from build123d import *

# Parameters (mm, degrees)
SKETCH1_R           = 25
SKETCH1_R_2         = 22.5
BOSS_EXTRUDE1_DEPTH = 130
SKETCH2_R           = 25
BOSS_EXTRUDE2_DEPTH = 5
BOSS_EXTRUDE3_DEPTH = 3
SKETCH4_R           = 2
BOSS_EXTRUDE4_DEPTH = 10


with BuildPart() as part:
    # Sketch1 → Boss-Extrude1 (new body)
    with BuildSketch(Plane(origin=(0, 0, 0), x_dir=(1, 0, 0), z_dir=(0, 1, 0))):
        Circle(SKETCH1_R)
        Circle(SKETCH1_R_2, mode=Mode.SUBTRACT)
    extrude(amount=BOSS_EXTRUDE1_DEPTH)

    # Sketch2 → Boss-Extrude2 (add)
    with BuildSketch(Plane.XZ):
        Circle(SKETCH2_R)
    extrude(amount=-BOSS_EXTRUDE2_DEPTH)

    # Sketch3 → Boss-Extrude3 (add)
    with BuildSketch(Plane(origin=(0, 130, 0), x_dir=(1, 0, 0), z_dir=(0, 1, 0))):
        with BuildLine():
            ThreePointArc((-2.5, 24.874685928), (-1.251569376, 24.968651828), (0, 25))
            Line((0, 25), (0, 40))
            Line((0, 40), (-2.5, 40))
            Line((-2.5, 40), (-2.5, 24.874685928))
        make_face()
        with BuildLine():
            Line((0, 40), (0, 25))
            ThreePointArc((0, 25), (1.251569376, 24.968651828), (2.5, 24.874685928))
            Line((2.5, 24.874685928), (2.5, 40))
            Line((2.5, 40), (0, 40))
        make_face()
    extrude(amount=-BOSS_EXTRUDE3_DEPTH)

    # Sketch4 → Boss-Extrude4 (add)
    with BuildSketch(Plane.XZ.offset(-127)):
        with Locations((0, -38)):
            Circle(SKETCH4_R)
    extrude(amount=BOSS_EXTRUDE4_DEPTH)


solid = part.part
Source: CAD feature listing. Evaluate the final solid. Frame: model axes, mm. A direction names the side the tool comes from. Give positions to 0.01 mm unless a question says otherwise; leave off trailing zeros. Write each loop counter-clockwise with the first axis right and the second up, starting at its lowest first coordinate (ties: lowest second). Pieces come first, ordered by that corner, then holes. Notation, with made-up numbers: M 45.25,59.5 L 74.25,59.5 A21 cw 74.25,96.5 Z; hole C 4,79.25 d5. An arc over 180 degrees is marked long. Return JSON: item names as keys, results as strings. Group by question number.
1) Cut plane C-C, the plane z = -27.5. Output: boundary loops of the cut face in (x, y), then the cut area to 3 significant figures.
2) Cut plane A-A, the plane z = 0. Output: boundary loops of the cut face in (x, y), then the cut area to 3 significant figures.
3) Set-up query: faces 4 (the face through (2.5, 129, -32)), 5 (the face through (0, 122, -40)), 6 (the face through (-2.5, 129, -33)), 7 (the face through (10.382, 66.625, 19.961)). Return all of +Z, -Z, +X, -X, +Y, -Y with unobstructed straight access to the full face (end or side cutting, diameter ignored); none if empty.
4) First-contact query: pin 1 Ø4.5 at (x, z) = (-1, -38.5) entering from -Y; pin 2 Ø5 at (x, z) = (-2, -10.5) entering from +Y; pin 3 Ø0.9 at (y, z) = (129, -35) entering from +X. Flat tips, straight axial feed; report the tip coordinate or a pass-through.
5) Draft query along Z for faces 1 (the face through (0, 127, -31)), 2 (the face through (0, 129, -40)), 3 (the face through (0, 117, -38)). Return one class per face: released by +Z, released by -Z, zero draft, split by the parting line, or undercut.
6) Cut plane B-B, the plane x = 4.5. Output: boundary loops of the cut face in (y, z), then the cut area to 3 significant figures.
7) Ray query, L1, parallel to X at y = 32, z = 0; L2, parallel to X at y = 96, z = -4. Return the intervals inside material, ascending.
Data:
{
 "1": {"outline": "M -2.5,127 L 2.5,127 L 2.5,130 L -2.5,130 Z", "area": "15.0 mm²"},
 "2": {"outline": "M -25,0 L 25,0 L 25,130 L 22.5,130 L 22.5,5 L -22.5,5 L -22.5,130 L -25,130 Z", "area": "875 mm²"},
 "3": {"face 4": "-Z, +X, +Y, -Y", "face 5": "-Y", "face 6": "-Z, -X, +Y, -Y", "face 7": "+Y"},
 "4": {"pin 1": "stops at y = 117", "pin 2": "stops at y = 5", "pin 3": "stops at x = 2.5"},
 "5": {"face 1": "undercut", "face 2": "released by -Z", "face 3": "zero draft"},
 "6": {"outline": "M 0,-24.59 L 130,-24.59 L 130,-22.05 L 5,-22.05 L 5,22.05 L 130,22.05 L 130,24.59 L 0,24.59 Z", "area": "882 mm²"},
 "7": {"L1": "x = -25 to -22.5, 22.5 to 25", "L2": "x = -24.68 to -22.14, 22.14 to 24.68"}
}
